```python
from build123d import *

# Parameters (mm, degrees)
F0_W      = 100
F0_H      = 100
F1_DEPTH  = 10
F2_W      = 5
F2_H      = 5
F3_DEPTH  = 100
F4_R      = 5
F5_R      = 2
F7_DEPTH  = 2
F8_SIZE   = 1
F9_W      = 10
F9_H      = 10
F10_DEPTH = 10


with BuildPart() as f1:
    # F0 (on Top) → F1 (new body)
    with BuildSketch(Plane.XY):
        Rectangle(F0_W, F0_H)
    extrude(amount=F1_DEPTH)

    # F2 (on face) → F3 (join)
    with BuildSketch(Plane(origin=(0, 0, 0), x_dir=(1, 0, 0), z_dir=(0, 0, -1))):
        with Locations((-42.5, 42.5)):
            Rectangle(F2_W, F2_H)
        with Locations((-42.5, -42.5)):
            Rectangle(F2_W, F2_H)
        with Locations((42.5, 42.5)):
            Rectangle(F2_W, F2_H)
        with Locations((42.5, -42.5)):
            Rectangle(F2_W, F2_H)
    extrude(amount=F3_DEPTH)

    # F4
    f4_edges = [f1.edges().sort_by_distance(p)[0] for p in [
        (0, 50, 10),
        (-50, 0, 10),
        (0, -50, 10),
        (50, 0, 10),
    ]]
    fillet(f4_edges, radius=F4_R)

    # F5
    f5_edges = [f1.edges().sort_by_distance(p)[0] for p in [
        (0, -50, 0),
        (50, 0, 0),
        (0, 50, 0),
        (-50, 0, 0),
    ]]
    fillet(f5_edges, radius=F5_R)

    # F6 (on face) → F7 (cut)
    with BuildSketch(Plane.XY.offset(10)):
        Polygon((-7.248737, -17.5), (7.248737, -17.5), (17.5, -7.248737), (17.5, 7.248737), (7.248737, 17.5), (-7.248737, 17.5), (-17.5, 7.248737), (-17.5, -7.248737), align=None)
    extrude(amount=-F7_DEPTH, mode=Mode.SUBTRACT)

    # F8
    f8_edges = [f1.edges().sort_by_distance(p)[0] for p in [
        (0, -17.5, 8),
        (12.374369, -12.374369, 8),
        (17.5, 0, 8),
        (12.374369, 12.374369, 8),
        (0, 17.5, 8),
        (-12.374369, 12.374369, 8),
        (-17.5, 0, 8),
        (-12.374369, -12.374369, 8),
    ]]
    chamfer(f8_edges, length=F8_SIZE)

    # F9 (on face) → F10 (cut, through all)
    with BuildSketch(Plane.XY.offset(10)):
        with Locations((35, 35)):
            Rectangle(F9_W, F9_H)
    extrude(amount=-F10_DEPTH, mode=Mode.SUBTRACT)


solid = f1.part
```
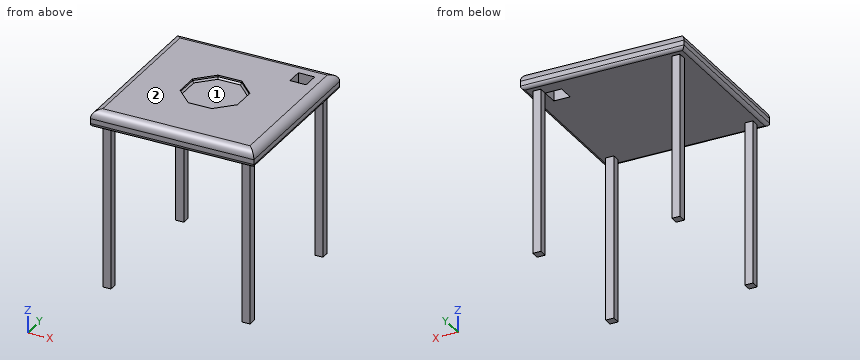
Source: CAD feature listing. Evaluate the final solid. Frame: model axes, mm. Face numbers are marked on the shaded views. Round coordinates to 2 decimals unless told otherwise and drop trailing zeros. Write each loop counter-clockwise with the first axis right and the second up, starting at its lowest first coordinate (ties: lowest second). Pieces come first, ordered by that corner, then holes. Notation, with made-up numbers: M -17,23.25 L 16,23.25 A29 ccw 16,60.25 Z; hole C 63,65 d11. An arc over 180 degrees is marked long. Answer as a JSON object with one key per item and string values. Group by question number.
(1) Mould query, pull axis Y, two halves, no side actions, for the marked faces 1 and 2. Classes: +Y half, -Y half, draft (parallel to the pull), parting line (faces both ways), or undercut.
(2) Section query B-B on z = -42.5. Output: boundary loops of the cut face in (x, y).
(3) First-contact query: pin 1 (5.5 mm diameter, centred on y = 42, z = -71, fed in from -X); pin 2 (4 mm diameter, centred on y = -42, z = -58.5, fed in from +X); pin 3 (5.5 mm diameter, centred on x = -41.5, z = -60.5, fed in from +Y); pin 4 (12 mm diameter, centred on y = -30.5, z = -76.5, fed in from -X). Flat tips, straight axial feed; report the tip coordinate or a pass-through.
(4) Section query A-A on y = 37.5. Output: boundary loops of the cut face in (x, z), then the cut area to 3 significant figures.
(5) Ray query, line 1 (X direction, y = -41, z = -71.5); line 2 (Z direction, x = 2, y = 13). Return the intervals inside material, ascending. Write a range as [from, to].
(6) Section query C-C on x = -33.5. Output: boundary loops of the cut face in (y, z).
Computed values:
{
 "1": {"face 1": "undercut", "face 2": "draft"},
 "2": {"outline": "M -45,-45 L -40,-45 L -40,-40 L -45,-40 Z; M -45,40 L -40,40 L -40,45 L -45,45 Z; M 40,-45 L 45,-45 L 45,-40 L 40,-40 Z; M 40,40 L 45,40 L 45,45 L 40,45 Z"},
 "3": {"pin 1": "x = -45", "pin 2": "x = 45", "pin 3": "y = 45", "pin 4": "through"},
 "4": {"outline": "M -50,2 A2 ccw -48,0 L 30,0 L 30,10 L -45,10 A5 ccw -50,5 Z; M 40,0 L 48,0 A2 ccw 50,2 L 50,5 A5 ccw 45,10 L 40,10 Z", "area": "888 mm^2"},
 "5": {"line 1": "[-45, -40], [40, 45]", "line 2": "[0, 8]"},
 "6": {"outline": "M -50,2 A2 ccw -48,0 L 48,0 A2 ccw 50,2 L 50,5 A5 ccw 45,10 L -45,10 A5 ccw -50,5 Z"}
}
